Check sheet for the modelled part. Datum: model origin and axes. Units: mm. A direction names the side the tool comes from. Give positions to 0.01 mm unless a question says otherwise; leave off trailing zeros. Loops run counter-clockwise (first coordinate to the right, second up) from the corner with the lowest first, then second, coordinate; pieces in that order, holes last. Notation, with made-up numbers: (0, -13.75) -> (19, -13.75) arc R30 cw to (19, 16.25) -> close; hole circle Ø1 at (26.25, -3.5). An arc over 180 degrees is marked (long way). Write each question's results on one line, items separated by ' | '. Start each with the question number.
1. Material ranges on L1, parallel to X at y = 9.5, z = 10; L2, parallel to X at y = 4, z = 7; L3, parallel to Y at x = 22, z = 10, recorded low to high. Write a range as from..to.
2. Mould release check, pull along Y, two halves, no side actions. Record for faces 4 (the face through (30.44, 15.13, 19.49)), 5 (the face through (25.22, 29.43, 19.4)), 6 (the face through (50, 15.2, 10.5)), 7 (the face through (25, 23, 10)): +Y half, -Y half, draft (parallel to the pull), parting line (faces both ways), or undercut.
3. Gauge pin test, flat ends, axial feed: pin 1 Ø2 at (y, z) = (12.5, 11.5) entering from -X; pin 2 Ø2 at (x, y) = (6, 8) entering from +Z; pin 3 Ø3 at (y, z) = (16, 16) entering from -X; pin 4 Ø3 at (y, z) = (12.5, 4.5) entering from +X. Record the tip position at first contact, or that the pin passes through.
4. Cross-section at C-C on y = 26. Record the boundary of the cut face in (x, z).
5. Cross-section at B-B on x = 22.5. Record the boundary of the cut face in (y, z), and give its area (3 significant figures).
6. Cross-section at D-D on z = 9. Count the separate pieces of the cut face and the enclosed holes in it, and give its area (3 significant figures).
7. Tool access check on faces 1 (the face through (19.951, 15, 10)), 2 (the face through (25, 6.5, 19.5)), 3 (the face through (18, 15, 0)). Record the directions out of +Z, -Z, +X, -X, +Y, -Y that give a thin tool (end or side, any length) a straight path to the whole face; none if there is none.
8. Cross-section at A-A on y = 20.75. Record the boundary of the cut face in (x, z).
Autodesk Fusion 360 part; units mm, degrees
box "Grundkörper Quader1" add length 30 width 50 height 20 placed x (0, 1, 0) y (-1, 0, 0) z (0, 0, 1) at (50, 0, 0)
sketch "Skizze2" plane through (0, 0, 0) normal (0, -1, 0) x (1, 0, 0)
  line L0 (0, 20) -> (0, 0)
  line L1 (0, 0) -> (50, 0)
  line L2 (50, 0) -> (50, 20)
  line L3 (50, 20) -> (0, 20)
sketch "Skizze3" plane through (0, 0, 0) normal (0, -1, 0) x (1, 0, 0)
  circle A0 centre (11, 10) radius 4.1
  circle A1 centre (39, 10) radius 4.1
  line L0 (0, 20) -> (0, 0)
  line L1 (50, 0) -> (50, 20)
  line L2 (50, 20) -> (0, 20)
  line L3 (50, 0) -> (0, 0)
  dimension "d6" = 8.2
  dimension "d7" = 8.2
  dimension "d8" = 28
  dimension "d10" = 11
  dimension "d11" = 10
  dimension "d23" = 10
hole "Bohrung1" at (11, 0, 10) direction (0, 1, 0) diameter 8.2 depth 30 tip angle 118
sketch "Skizze4" plane through (0, 0, 0) normal (0, -1, 0) x (1, 0, 0)
hole "Bohrung2" at (39, 0, 10) direction (0, 1, 0) diameter 8.2 depth 30 tip angle 118
fillet "Abrundung1" radius 9 2 edges at (0, 15, 20) (50, 15, 20)
fillet "Abrundung2" radius 10 2 edges at (50, 15, 0) (0, 15, 0)
fillet "Abrundung3" radius 2 8 edges at (50, 0, 10.5) (47.0711, 0, 2.9289) (25, 0, 0) (2.9289, 0, 2.9289) (0, 0, 10.5) (2.636, 0, 17.364) (25, 0, 20) (47.364, 0, 17.364)
fillet "Abrundung4" radius 2 8 edges at (0, 30, 10.5) (2.9289, 30, 2.9289) (25, 30, 0) (47.0711, 30, 2.9289) (50, 30, 10.5) (47.364, 30, 17.364) (25, 30, 20) (2.636, 30, 17.364)
chamfer "Fase1" distance 2 angle 45 2 edges at (37.5174, 30, 13.8225) (9.5174, 30, 13.8225)
chamfer "Fase2" distance 2 angle 45 2 edges at (12.4826, 0, 13.8225) (40.4826, 0, 13.8225)
sketch "Skizze5" plane through (0, 0, 20) normal (0, 0, 1) x (-1, 0, 0)
  line L0 (-41, -28) -> (-9, -28)
  line L1 (-9, -28) -> (-9, -2)
  line L2 (-9, -2) -> (-41, -2)
  line L3 (-41, -2) -> (-41, -28)
  line L4 (-29.951, -7) -> (-29.951, -23)
  line L5 (-29.951, -23) -> (-19.951, -23)
  line L6 (-19.951, -23) -> (-19.951, -7)
  line L7 (-19.951, -7) -> (-29.951, -7)
extrude "Extrusion1" cut sketch "Skizze5" against normal blind 32 contours L4 L5 L6 L7
chamfer "Fase3" distance 1 angle 45 4 edges at (19.951, 15, 20) (29.951, 15, 20) (24.951, 7, 20) (24.951, 23, 20)
Geometry says:
1) L1: 0..6.9, 15.1..19.95, 29.95..34.9, 43.1..50 | L2: 0.46..8.21, 13.79..36.21, 41.79..49.54 | L3: 0..7, 23..30
2) face 4: undercut | face 5: +Y half | face 6: draft | face 7: undercut
3) pin 1: x = 0 | pin 2: z = 19.77 | pin 3: x = 0.71 | pin 4: x = 49.17
4) outline: (0, 10) arc R10 ccw to (10, 0) -> (40, 0) arc R10 ccw to (50, 10) -> (50, 11) arc R9 ccw to (41, 20) -> (9, 20) arc R9 ccw to (0, 11) -> close; hole circle Ø8.2 at (11, 10); hole circle Ø8.2 at (39, 10)
5) outline: (0, 2) arc R2 ccw to (2, 0) -> (7, 0) -> (7, 19) -> (6, 20) -> (2, 20) arc R2 ccw to (0, 18) -> close; (23, 0) -> (28, 0) arc R2 ccw to (30, 2) -> (30, 18) arc R2 ccw to (28, 20) -> (24, 20) -> (23, 19) -> close | area: 276 mm^2
6) separate pieces: 3 | enclosed holes: 1 | area: 840 mm^2
7) face 1: +Z, -Z | face 2: +Z | face 3: -Z, +X, -X, +Y, -Y
8) outline: (0, 10) arc R10 ccw to (10, 0) -> (19.95, 0) -> (19.95, 19) -> (18.95, 20) -> (9, 20) arc R9 ccw to (0, 11) -> close; (29.95, 0) -> (40, 0) arc R10 ccw to (50, 10) -> (50, 11) arc R9 ccw to (41, 20) -> (30.95, 20) -> (29.95, 19) -> close; hole circle Ø8.2 at (11, 10); hole circle Ø8.2 at (39, 10)
